For this review, use the dimensioned drawing (mm, ordinates from the lowest corner) and the shaded views. A direction names the side the tool comes from. Coordinates: 2 decimals unless noted, no trailing zeros. Write each loop counter-clockwise with the first axis right and the second up, starting at its lowest first coordinate (ties: lowest second). Pieces come first, ordered by that corner, then holes. Notation, with made-up numbers: M -11,-38.5 L 27,-38.5 A28 cw 27,-4.5 Z; hole C 36,59 d1. An arc over 180 degrees is marked long. One line per question, with ' | ' between items.
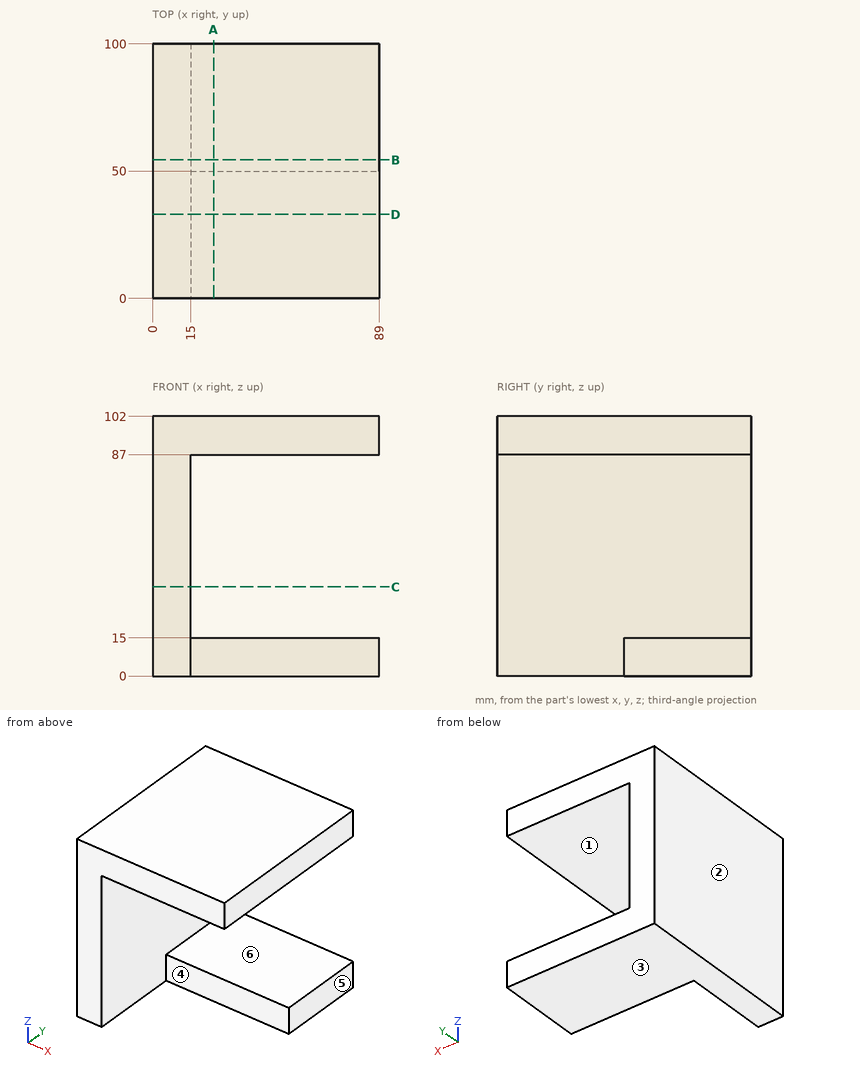
1. Insertion check: pin 1 Ø16.5 at (x, z) = (70.5, 6) entering from -Y; pin 2 Ø1.5 at (x, y) = (63, 25) entering from -Z. Each pin has a flat end and moves straight along its axis. Give the tip position at first contact, or say it passes through.
Answer sheet:
pin 1: y = 50 | pin 2: z = 87
2. Take a section at B-B (y = 54.5). Write out the cut boundary in (x, z), then the cut area to 3 significant figures.
Answer sheet:
outline: M 0,0 L 89,0 L 89,15 L 15,15 L 15,87 L 89,87 L 89,102 L 0,102 Z | area: 3,750 mm^2
3. Take a section at D-D (y = 33). Write out the cut boundary in (x, z), then the cut area to 3 significant figures.
Answer sheet:
outline: M 0,0 L 15,0 L 15,87 L 89,87 L 89,102 L 0,102 Z | area: 2,640 mm^2
4. Tool access review of the marked faces 4, 5 and 6: name each direction out of +Z, -Z, +X, -X, +Y, -Y from which nothing blocks a thin tool from reaching the whole face with its end or side.
Answer sheet:
face 4: -Z, +X, -Y | face 5: +Z, -Z, +X, +Y, -Y | face 6: +X, +Y, -Y
5. To check wall thickness, follow line 1 along Z through (x, y) = (48.5, 78); line 2 along X through (y, z) = (41, 56.5); line 3 along Y through (x, z) = (48, 11.5). State the ranges of each line that lie inside material, in increasing order. Write a range as [from, to].
Answer sheet:
line 1: [0, 15], [87, 102] | line 2: [0, 15] | line 3: [50, 100]
6. Take a section at C-C (z = 35). Write out the cut boundary in (x, y), then the cut area to 3 significant figures.
Answer sheet:
outline: M 0,0 L 15,0 L 15,100 L 0,100 Z | area: 1,500 mm^2
7. Take a section at A-A (x = 24). Write out the cut boundary in (y, z), then the cut area to 3 significant figures.
Answer sheet:
outline: M 0,87 L 100,87 L 100,102 L 0,102 Z; M 50,0 L 100,0 L 100,15 L 50,15 Z | area: 2,250 mm^2
8. Draft analysis for pull direction Z (two halves, no side actions). For the marked faces 1, 2 and 3, state which applies: pulls with the +Z half, pulls with the -Z half, needs draft (parallel to the pull), parting line crosses it, or undercut.
Answer sheet:
face 1: undercut | face 2: needs draft | face 3: pulls with the -Z half
